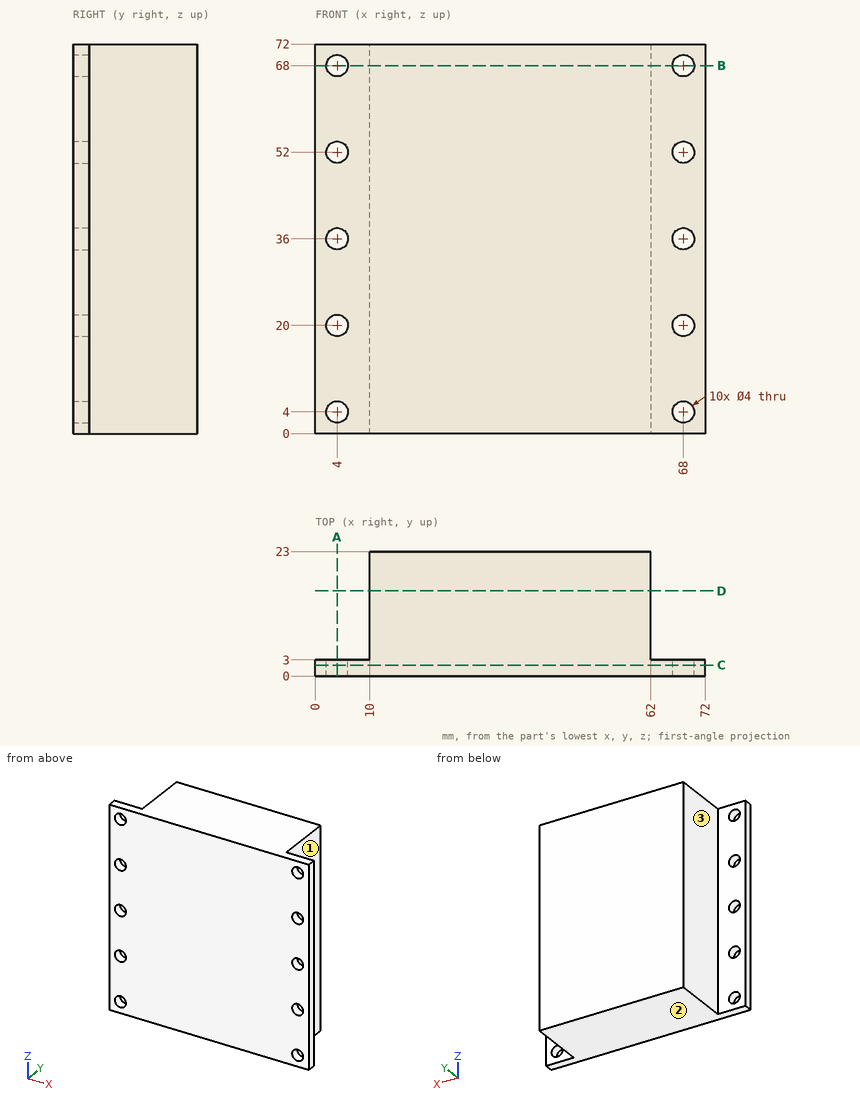
Study the drawing (mm; zero at the part's minimum x, y, z) and answer. A direction names the side the tool comes from. Give positions to 0.01 mm unless a question says otherwise; leave off trailing zeros. Write each loop counter-clockwise with the first axis right and the second up, starting at its lowest first coordinate (ties: lowest second). Pieces come first, ordered by that corner, then holes. Notation, with made-up numbers: (8, -35.75) -> (25, -35.75) arc R25 cw to (25, -17.75) -> close; hole circle Ø7 at (44.5, 56.25). An arc over 180 degrees is marked (long way). Write item = value, one per line.
Q1. A tool of negligible diameter and unlimited length cuts with its end or side. For the marked faces 1, 2 and 3, from which of +Z, -Z, +X, -X, +Y, -Y can it reach the whole face along a straight path? Write none if from no direction.
Computed values:
face_1 = +Z, -Z, +X, +Y
face_2 = -Z, +X, -X, +Y, -Y
face_3 = +Z, -Z, -X, +Y
Q2. Section A-A on x = 4 is taken. Determine the outline of the cut face in (y, z), and give its area (3 significant figures).
Computed values:
outline = (0, 0) -> (3, 0) -> (3, 2) -> (0, 2) -> close; (0, 6) -> (3, 6) -> (3, 18) -> (0, 18) -> close; (0, 22) -> (3, 22) -> (3, 34) -> (0, 34) -> close; (0, 38) -> (3, 38) -> (3, 50) -> (0, 50) -> close; (0, 54) -> (3, 54) -> (3, 66) -> (0, 66) -> close; (0, 70) -> (3, 70) -> (3, 72) -> (0, 72) -> close
area = 156 mm^2
Q3. Section B-B on z = 68 is taken. Determine the outline of the cut face in (x, y).
Computed values:
outline = (0, 0) -> (2, 0) -> (2, 3) -> (0, 3) -> close; (6, 0) -> (66, 0) -> (66, 3) -> (62, 3) -> (62, 23) -> (10, 23) -> (10, 3) -> (6, 3) -> close; (70, 0) -> (72, 0) -> (72, 3) -> (70, 3) -> close
Q4. Flat-ended cylindrical pins translate along their axes: pin 1 Ø2.5 at (x, z) = (68, 4) entering from -Y; pin 2 Ø1.5 at (x, y) = (14, 3) entering from -Z; pin 3 Ø6 at (y, z) = (10, 54) entering from +X; pin 4 Ø8 at (x, z) = (3.5, 30.5) entering from +Y. Find the tip coordinate at first contact, or state that the pin passes through.
Computed values:
pin_1 = through
pin_2 = 0
pin_3 = 62
pin_4 = 3
Q5. Section D-D on y = 15.75 is taken. Determine the outline of the cut face in (x, z), and give its area (3 significant figures).
Computed values:
outline = (10, 0) -> (62, 0) -> (62, 72) -> (10, 72) -> close
area = 3,740 mm^2
Q6. Section C-C on y = 2 is taken. State how many separate pieces and enclosed holes the cut face has, and give its area (3 significant figures).
Computed values:
separate_pieces = 1
enclosed_holes = 10
area = 5,060 mm^2
Q7. Consider line 1 along X through (y, z) = (1.1, 20); line 2 along Z through (x, y) = (68, 1); line 3 along X through (y, z) = (14, 59). Determine where each line is inside the solid, lowest interval first.
Computed values:
line_1 = 0 to 2, 6 to 66, 70 to 72
line_2 = 0 to 2, 6 to 18, 22 to 34, 38 to 50, 54 to 66, 70 to 72
line_3 = 10 to 62
